```python
from build123d import *

# Parameters (mm, degrees)
F1_DEPTH = 0.7
F2_R     = 4.5
F3_DEPTH = 2
F5_DEPTH = 10
F6_R     = 8
F7_DEPTH = 4.5
F8_R     = 19.5
F9_DEPTH = 2


with BuildPart() as f1:
    # F0 (on Top) → F1 (new body)
    with BuildSketch(Plane.XY):
        Polygon((-12.9903810568, -22.5), (12.9903810568, -22.5), (25.9807621135, 0), (12.9903810568, 22.5), (-12.9903810568, 22.5), (-25.9807621135, 0), align=None)
    extrude(amount=F1_DEPTH)

    # F2 (on face) → F3 (join)
    with BuildSketch(Plane.XY.offset(0.7)):
        Polygon((-12.9903810568, 22.5), (-25.9807621135, 0), (-12.9903810568, -22.5), (12.9903810568, -22.5), (25.9807621135, 0), (12.9903810568, 22.5), align=None)
        Circle(F2_R, mode=Mode.SUBTRACT)
    extrude(amount=F3_DEPTH)

    # F4 (on face) → F5 (join)
    with BuildSketch(Plane.XY.offset(2.7)):
        Polygon((12.9903810568, -22.5), (25.9807621135, 0), (12.9903810568, 22.5), (-12.9903810568, 22.5), (-25.9807621135, 0), (-12.9903810568, -22.5), align=None)
        Polygon((7.7942286341, 0), (3.897114317, -6.75), (-3.897114317, -6.75), (-7.7942286341, 0), (-3.897114317, 6.75), (3.897114317, 6.75), align=None, mode=Mode.SUBTRACT)
    extrude(amount=F5_DEPTH)

    # F6 (on face) → F7 (join)
    with BuildSketch(Plane.XY.offset(12.7)):
        Polygon((-12.9903810568, -22.5), (12.9903810568, -22.5), (25.9807621135, 0), (12.9903810568, 22.5), (-12.9903810568, 22.5), (-25.9807621135, 0), align=None)
        Circle(F6_R, mode=Mode.SUBTRACT)
    extrude(amount=F7_DEPTH)

    # F8 (on face) → F9 (join)
    with BuildSketch(Plane.XY.offset(17.2)):
        Polygon((-12.9903810568, 22.5), (-25.9807621135, 0), (-12.9903810568, -22.5), (12.9903810568, -22.5), (25.9807621135, 0), (12.9903810568, 22.5), align=None)
        Circle(F8_R, mode=Mode.SUBTRACT)
    extrude(amount=F9_DEPTH)


solid = f1.part
```
Here's how the part is built. I have some questions about the finished solid (model axes, mm). A direction names the side the tool comes from. Coordinates: 2 decimals unless noted, no trailing zeros. Loops run counter-clockwise (first coordinate to the right, second up) from the corner with the lowest first, then second, coordinate; pieces in that order, holes last. Notation, with made-up numbers: (46, 8) - (62, 8) arc R19 ccw to (62, 14) - close; hole circle Ø4 at (-38.5, 55.25). An arc over 180 degrees is marked (long way). Return JSON: item names as keys, results as strings. Group by question number.
Item 1: Will these pins go through, and if not, where does the flat tip stop? P1, Ø11.5, axis at x = 0.5, y = 5, coming from the +Z side; P2, Ø10, axis at x = -0.5, y = 1.5, coming from the +Z side; P3, Ø1.5, axis at y = 2.5, z = 7, coming from the -X side.
Item 2: On a 3-axis mill with a long thin cutter (end or side, diameter ignored), from which of +Z, -Z, +X, -X, +Y, -Y can I reach the whole of each face in a straight line? I mean faces 1 (the face through (0, 22.5, 9)), 2 (the face through (-1.73, -7.81, 14.92)). Say none if no direction works.
Item 3: If we section it at C-C on y = -10.5: Write out the boundary of the cut face in (x, z), and give its area (3 significant figures).
Item 4: I need wall thicknesses on line 1 (Y direction, x = 0, z = 14.65); line 2 (Y direction, x = 0, z = 18.7); line 3 (Z direction, x = -13.5, y = 13). Which ranges of each line are inside material? Lowest first, please. Write a range as from..to.
Item 5: We'd pull the mould along Y, two halves only. Please class faces 3 (the face through (0, -22.5, 9)), 4 (the face through (-5.87, 3.33, 7.63)), 5 (the face through (0, 0, 0)): +Y half, -Y half, draft (parallel to the pull), parting line (faces both ways), or undercut.
Item 6: If we section it at A-A on z = 6: Write out the boundary of the cut face in (x, y).
Item 7: If we section it at B-B on x = 0: Write out the boundary of the cut face in (y, z), and give its area (3 significant figures).
Item 8: If we section it at D-D on z = 2: Write out the boundary of the cut face in (x, y), and give its area (3 significant figures).
Calculated:
{
 "1": {"P1": "stops at z = 17.2", "P2": "stops at z = 2.7", "P3": "stops at x = -24.97"},
 "2": {"face 1": "+Z, -Z, +X, -X, +Y", "face 2": "+Z"},
 "3": {"outline": "(-19.92, 0) - (19.92, 0) - (19.92, 19.2) - (16.43, 19.2) - (16.43, 17.2) - (-16.43, 17.2) - (-16.43, 19.2) - (-19.92, 19.2) - close", "area": "699 mm^2"},
 "4": {"line 1": "y = -22.5..-8, 8..22.5", "line 2": "y = -22.5..-19.5, 19.5..22.5", "line 3": "z = 0..17.2"},
 "5": {"face 3": "-Y half", "face 4": "undercut", "face 5": "draft"},
 "6": {"outline": "(-25.98, 0) - (-12.99, -22.5) - (12.99, -22.5) - (25.98, 0) - (12.99, 22.5) - (-12.99, 22.5) - close; hole (-7.79, 0) - (-3.9, -6.75) - (3.9, -6.75) - (7.79, 0) - (3.9, 6.75) - (-3.9, 6.75) - close"},
 "7": {"outline": "(-22.5, 0) - (22.5, 0) - (22.5, 19.2) - (19.5, 19.2) - (19.5, 17.2) - (8, 17.2) - (8, 12.7) - (6.75, 12.7) - (6.75, 2.7) - (4.5, 2.7) - (4.5, 0.7) - (-4.5, 0.7) - (-4.5, 2.7) - (-6.75, 2.7) - (-6.75, 12.7) - (-8, 12.7) - (-8, 17.2) - (-19.5, 17.2) - (-19.5, 19.2) - (-22.5, 19.2) - close", "area": "561 mm^2"},
 "8": {"outline": "(-25.98, 0) - (-12.99, -22.5) - (12.99, -22.5) - (25.98, 0) - (12.99, 22.5) - (-12.99, 22.5) - close; hole circle Ø9 at (0, 0)", "area": "1,690 mm^2"}
}
